Input: part model. Units: mm. Frame: model coordinates. A direction names the side the tool comes from. Round coordinates to 2 decimals unless told otherwise and drop trailing zeros. Order: outer loops, then holes, each group sorted by start corner. A loop starts at its lowest first (then second) coordinate and runs counter-clockwise, first axis right, second up. Notation, with made-up numbers: (85.25, -27.75) -> (140.25, -27.75) arc R5 cw to (140.25, -18.75) -> close; hole circle Ø9 at (67, 32). An arc over 180 degrees is marked (long way). Use a Markdown table: item, result.
from build123d import *

# Parameters (mm, degrees)
SKETCH1_W           = 20.1
SKETCH1_H           = 4.2
BOSS_EXTRUDE1_DEPTH = 4
SKETCH2_R           = 0.8
CUT_EXTRUDE1_DEPTH  = 4
SKETCH2_3_R         = 0.8
CUT_EXTRUDE2_DEPTH  = 4
LPATTERN1_COUNT     = 6
LPATTERN1_PITCH     = 25
LPATTERN2_COUNT     = 4
LPATTERN2_PITCH     = 25


with BuildPart() as part:
    # Sketch1 → Boss-Extrude1 (new body)
    with BuildSketch(Plane.XY):
        Polygon((-63.114700901, 60), (-63.114700901, -60), (-44.114700901, -60), (15.164047805, -32.5), (15.164047805, -28.3), (35.1, -28.3), (35.1, -32.5), (45.885299099, -32.5), (45.885299099, -26.3), (41.685299099, -26.3), (41.685299099, -6.2), (45.885299099, -6.2), (45.885299099, -8.64710736), (45.885299099, -18.248106547), (60.000337735, -11.7), (60.000337735, 11.7), (-44.114700901, 60), align=None)
        with Locations((-25.05, -30.4)):
            Rectangle(SKETCH1_W, SKETCH1_H, mode=Mode.SUBTRACT)
        with Locations((25.05, 9.6)):
            Rectangle(SKETCH1_W, SKETCH1_H, mode=Mode.SUBTRACT)
        with Locations((-25.05, 9.6)):
            Rectangle(SKETCH1_W, SKETCH1_H, mode=Mode.SUBTRACT)
    extrude(amount=BOSS_EXTRUDE1_DEPTH)

    # Sketch2 → Cut-Extrude1 (cut)
    with BuildSketch(Plane.XY.offset(4)):
        with Locations((-53.614700901, 50)):
            Circle(SKETCH2_R)
    cut_extrude1 = extrude(amount=-CUT_EXTRUDE1_DEPTH, mode=Mode.SUBTRACT)

    # Sketch2<3> → Cut-Extrude2 (cut)
    with BuildSketch(Plane.XY.offset(4)):
        with Locations((50.000337735, 0)):
            Circle(SKETCH2_3_R)
    cut_extrude2 = extrude(amount=-CUT_EXTRUDE2_DEPTH, mode=Mode.SUBTRACT)

    # LPattern1: Cut-Extrude1 ×6
    with Locations(*[(0, -i * LPATTERN1_PITCH, 0) for i in range(1, LPATTERN1_COUNT)]):
        add(cut_extrude1, mode=Mode.SUBTRACT)

    # LPattern2: Cut-Extrude2 ×4
    with Locations(*[(-i * LPATTERN2_PITCH, 0, 0) for i in range(1, LPATTERN2_COUNT)]):
        add(cut_extrude2, mode=Mode.SUBTRACT)


solid = part.part
1) Cut plane B-B on z = 1.45. State how many separate pieces and enclosed holes the cut face has, and give its area (3 significant figures).
Answer key:
| item | result |
|---|---|
| separate pieces | 1 |
| enclosed holes | 12 |
| area | 9,520 mm^2 |
2) Cut plane D-D on x = -12.5. Return loops of the section in (y, z), and give its area (3 significant figures).
Answer key:
| item | result |
|---|---|
| outline | (-45.33, 0) -> (45.33, 0) -> (45.33, 4) -> (-45.33, 4) -> close |
| area | 363 mm^2 |
3) Set-up query: faces 4 (the face through (-25, -32.5, 2)), 5 (the face through (40, -32.5, 2)), 6 (the face through (25, -28.3, 2)). Return all of +Z, -Z, +X, -X, +Y, -Y with unobstructed straight access to the full face (end or side cutting, diameter ignored); none if empty.
Answer key:
| item | result |
|---|---|
| face 4 | +Z, -Z |
| face 5 | +Z, -Z, +X, -Y |
| face 6 | +Z, -Z, -Y |
4) Ray query, probe 1 along Y at (x, z) = (-29.5, 0.3); probe 2 along Y at (x, z) = (-25, 0.95); probe 3 along X at (y, z) = (-21, 0.85). Return the intervals inside material, ascending.
Answer key:
| item | result |
|---|---|
| probe 1 | y = -53.22 to -32.5, -28.3 to 7.5, 11.7 to 53.22 |
| probe 2 | y = -51.13 to -32.5, -28.3 to -0.8, 0.8 to 7.5, 11.7 to 51.13 |
| probe 3 | x = -63.11 to 41.69 |
5) Cut plane C-C on y = -42.5. Return loops of the section in (x, z).
Answer key:
| item | result |
|---|---|
| outline | (-63.11, 0) -> (-6.39, 0) -> (-6.39, 4) -> (-63.11, 4) -> close |
6) Cut plane A-A on x = -28. Return loops of the section in (y, z), and give its area (3 significant figures).
Answer key:
| item | result |
|---|---|
| outline | (-52.52, 0) -> (-32.5, 0) -> (-32.5, 4) -> (-52.52, 4) -> close; (-28.3, 0) -> (7.5, 0) -> (7.5, 4) -> (-28.3, 4) -> close; (11.7, 0) -> (52.52, 0) -> (52.52, 4) -> (11.7, 4) -> close |
| area | 387 mm^2 |
7) Draft query along X for faces 1 (the face through (-15, 10, 2)), 2 (the face through (44, -26.3, 2)), 3 (the face through (45.885, -29, 2)). Return one class per face: released by +X, released by -X, zero draft, split by the parting line, or undercut.
Answer key:
| item | result |
|---|---|
| face 1 | undercut |
| face 2 | zero draft |
| face 3 | released by +X |
8) Contact query for flat-ended pins moving along their axis: P1, Ø1.2, axis at x = 43.5, z = 1, coming from the -Y side; P2, Ø2, axis at x = -38, z = 0.5, coming from the +Y side; P3, Ø2, axis at x = -21, z = 2.5, coming from the +Y side. Output: stop coordinate, or through.
Answer key:
| item | result |
|---|---|
| P1 | stops at y = -32.5 |
| P2 | stops at y = 57.63 |
| P3 | stops at y = 49.74 |
